from build123d import *

# Parameters (mm, degrees)
SKETCH009_W     = 56
SKETCH009_H     = 120.5
PAD004_DEPTH    = 20.5
SKETCH010_W     = 52
SKETCH010_H     = 53
SKETCH010_H_2   = 62
POCKET005_DEPTH = 18.5
POCKET006_DEPTH = 289.39875
FILLET005_R     = 1
FILLET006_R     = 0.5


with BuildPart() as part:
    # Sketch009 → Pad004 (new body)
    with BuildSketch(Plane.XY):
        Rectangle(SKETCH009_W, SKETCH009_H)
    extrude(amount=PAD004_DEPTH)

    # Sketch010 (on DatumPlane) → Pocket005 (cut)
    with BuildSketch(Plane(origin=(0, 4.5, 20.5), x_dir=(1, 0, 0), z_dir=(0, 0, 1))):
        with Locations((0, 27.25)):
            Rectangle(SKETCH010_W, SKETCH010_H)
        with Locations((0, -31.75)):
            Rectangle(SKETCH010_W, SKETCH010_H_2)
    extrude(amount=-POCKET005_DEPTH, mode=Mode.SUBTRACT)

    # Sketch011 (on DatumPlane) → Pocket006 (cut, through all)
    with BuildSketch(Plane(origin=(20, 0, 20.5), x_dir=(1, 0, 0), z_dir=(0, 0, 1))):
        with BuildLine():
            Line((0, 41.75), (30, 41.75))
            Line((30, 41.75), (30, 21.75))
            Line((30, 21.75), (0, 21.75))
            ThreePointArc((0, 41.75), (-10, 31.75), (0, 21.75))
        make_face()
        with BuildLine():
            Line((0, -17.25), (30, -17.25))
            Line((30, -17.25), (30, -37.25))
            Line((30, -37.25), (0, -37.25))
            ThreePointArc((0, -17.25), (-10, -27.25), (0, -37.25))
        make_face()
    pocket006 = extrude(amount=-POCKET006_DEPTH, mode=Mode.SUBTRACT)

    # Mirrored003: Pocket006 across YZ
    add(pocket006.mirror(Plane.YZ), mode=Mode.SUBTRACT)

    # Fillet005
    fillet005_edges = [part.edges().sort_by_distance(p)[0] for p in [
        (0, 60.25, 0),
        (28, 51, 0),
        (24, 41.75, 0),
        (10, 31.75, 0),
        (24, 21.75, 0),
        (28, 2.25, 0),
        (24, -17.25, 0),
        (10, -27.25, 0),
        (24, -37.25, 0),
        (28, -48.75, 0),
        (0, -60.25, 0),
        (-28, -48.75, 0),
        (-24, -37.25, 0),
        (-10, -27.25, 0),
        (-24, -17.25, 0),
        (-28, 2.25, 0),
        (-24, 21.75, 0),
        (-10, 31.75, 0),
        (-24, 41.75, 0),
        (-28, 51, 0),
    ]]
    fillet(fillet005_edges, radius=FILLET005_R)

    # Fillet006
    fillet006_edges = [part.edges().sort_by_distance(p)[0] for p in [
        (0, 60.25, 20.5),
        (28, 51, 20.5),
        (27, 41.75, 20.5),
        (26, 50, 20.5),
        (0, 58.25, 20.5),
        (-26, 50, 20.5),
        (-27, 41.75, 20.5),
        (-28, 51, 20.5),
        (-27, 21.75, 20.5),
        (-26, 13.5, 20.5),
        (0, 5.25, 20.5),
        (26, 13.5, 20.5),
        (27, 21.75, 20.5),
        (28, 2.25, 20.5),
        (27, -17.25, 20.5),
        (26, -6.75, 20.5),
        (0, 3.75, 20.5),
        (-26, -6.75, 20.5),
        (-27, -17.25, 20.5),
        (-28, 2.25, 20.5),
        (-27, -37.25, 20.5),
        (-26, -47.75, 20.5),
        (0, -58.25, 20.5),
        (26, -47.75, 20.5),
        (27, -37.25, 20.5),
        (28, -48.75, 20.5),
        (0, -60.25, 20.5),
        (-28, -48.75, 20.5),
    ]]
    fillet(fillet006_edges, radius=FILLET006_R)


with BuildPart() as part_1:
    # Body003 placement: moved
    add(part.part.moved(Location((-67, 84, 14))))


solid = part_1.part
Input: part model. Units: mm. Frame: model coordinates. A direction names the side the tool comes from. Round coordinates to 2 decimals unless told otherwise and drop trailing zeros. Order: outer loops, then holes, each group sorted by start corner. A loop starts at its lowest first (then second) coordinate and runs counter-clockwise, first axis right, second up. Notation, with made-up numbers: (-9, -14) - (16, -14) arc R23 ccw to (16, 22) - close; hole circle Ø5 at (89, 65.5). An arc over 180 degrees is marked (long way). Answer as a JSON object with one key per item and string values. Group by question number.
(1) Pin query (flat end, axial travel): P1, Ø4, axis at x = -61, y = 67, coming from the +Z side. Return the tip coordinate at first contact, or that it passes through.
(2) Cut plane D-D (y = 135). Return loops of the section in (x, z).
(3) Draft query along X for faces 5 (the face through (-94, 86, 34.5)), 6 (the face through (-93, 36, 25)), 7 (the face through (-95, 135, 24)). Return one class per face: released by +X, released by -X, zero draft, split by the parting line, or undercut.
(4) Material intervals for probe 1 along Y at (x, z) = (-90, 17.25); probe 2 along X at (y, z) = (82, 21); probe 3 along Z at (x, y) = (-77, 133), sorted ascending. Write a range as from..to.
(5) Cut plane C-C (y = 56.75). Return loops of the section in (x, z), then the cut area to 3 significant figures.
(6) Cut plane B-B (x = -73). Return loops of the section in (y, z), then the cut area to 3 significant figures.
(7) Reachability of faces 1 (the face through (-39, 86, 24)), 2 (the face through (-40.6, 105.75, 23.8)), 3 (the face through (-93.4, 105.75, 23.8)), 4 (the face through (-41, 36, 25)) from +Z, -Z, +X, -X, +Y, -Y: full face, straight path, thin tool, end or side. Return the list, or none.
(8) Cut plane A-A (z = 32.75). Return loops of the section in (x, y).
Here are the results:
{
 "1": {"P1": "stops at z = 16"},
 "2": {"outline": "(-95, 15) arc R1 ccw to (-94, 14) - (-40, 14) arc R1 ccw to (-39, 15) - (-39, 34) arc R0.5 ccw to (-39.5, 34.5) - (-40.5, 34.5) arc R0.5 ccw to (-41, 34) - (-41, 16) - (-93, 16) - (-93, 34) arc R0.5 ccw to (-93.5, 34.5) - (-94.5, 34.5) arc R0.5 ccw to (-95, 34) - close"},
 "3": {"face 5": "zero draft", "face 6": "undercut", "face 7": "released by -X"},
 "4": {"probe 1": "y = 23.75..25.75, 87.75..89.25, 142.25..144.25", "probe 2": "x = -95..-93, -41..-39", "probe 3": "z = 14..16"},
 "5": {"outline": "(-77, 15) arc R1 ccw to (-76, 14) - (-58, 14) arc R1 ccw to (-57, 15) - (-57, 16) - (-77, 16) - close", "area": "39.6 mm^2"},
 "6": {"outline": "(23.75, 15) arc R1 ccw to (24.75, 14) - (143.25, 14) arc R1 ccw to (144.25, 15) - (144.25, 34) arc R0.5 ccw to (143.75, 34.5) - (142.75, 34.5) arc R0.5 ccw to (142.25, 34) - (142.25, 16) - (89.25, 16) - (89.25, 34) arc R0.5 ccw to (88.75, 34.5) - (88.25, 34.5) arc R0.5 ccw to (87.75, 34) - (87.75, 16) - (25.75, 16) - (25.75, 34) arc R0.5 ccw to (25.25, 34.5) - (24.25, 34.5) arc R0.5 ccw to (23.75, 34) - close", "area": "342 mm^2"},
 "7": {"face 1": "+Z, -Z, +X, +Y, -Y", "face 2": "+Z, -Z, +X", "face 3": "+Z, -Z, -X", "face 4": "+Z"},
 "8": {"outline": "(-95, 23.75) - (-39, 23.75) - (-39, 46.75) - (-41, 46.75) - (-41, 25.75) - (-93, 25.75) - (-93, 46.75) - (-95, 46.75) - close; (-95, 66.75) - (-93, 66.75) - (-93, 87.75) - (-41, 87.75) - (-41, 66.75) - (-39, 66.75) - (-39, 105.75) - (-41, 105.75) - (-41, 89.25) - (-93, 89.25) - (-93, 105.75) - (-95, 105.75) - close; (-95, 125.75) - (-93, 125.75) - (-93, 142.25) - (-41, 142.25) - (-41, 125.75) - (-39, 125.75) - (-39, 144.25) - (-95, 144.25) - close"}
}
